Model file for the job. Use its own axes, mm. Face numbers are marked on the shaded views. A direction names the side the tool comes from. Round coordinates to 2 decimals unless told otherwise and drop trailing zeros. One line per item, written item: value.
from build123d import *

# Parameters (mm, degrees)
SKETCH1_R            = 4.1
BOSS_EXTRUDE1_DEPTH  = 6.35
SKETCH4_R            = 2
BOSS_EXTRUDE2_DEPTH  = 3
SKETCH6_R            = 1.999996081
BOSS_EXTRUDE4_DEPTH  = 3
SKETCH8_R            = 1.999996
BOSS_EXTRUDE5_DEPTH  = 3
SKETCH9_R            = 1.999996
BOSS_EXTRUDE6_DEPTH  = 3
SKETCH10_R           = 1.999996
BOSS_EXTRUDE7_DEPTH  = 3
SKETCH11_R           = 1.999996
BOSS_EXTRUDE8_DEPTH  = 3
SKETCH12_R           = 2.5
BOSS_EXTRUDE9_DEPTH  = 25.4
SKETCH15_R           = 5.5
SKETCH15_R_2         = 4
BOSS_EXTRUDE10_DEPTH = 2.54


with BuildPart() as part:
    # Sketch1 → Boss-Extrude1 (new body)
    with BuildSketch(Plane(origin=(0, 0, 0), x_dir=(1, 0, 0), z_dir=(0, 1, 0))):
        Polygon((1.878116929, -32.317100962), (-12.817952122, -29.725787478), (-10.907822168, -18.892902195), (3.788246884, -21.484215679), align=None)
        Polygon((-10.907822168, -18.892902195), (3.788246884, -21.484215679), (16.711753116, -14.022825876), (21.815644336, 0), (16.711753116, 14.022825876), (3.788246884, 21.484215679), (-10.907822168, 18.892902195), (-20.5, 7.461389802), (-20.5, -7.461389802), align=None)
        Circle(SKETCH1_R, mode=Mode.SUBTRACT)
        Polygon((27.048371945, 17.785047453), (32.152263164, 3.762221577), (21.815644336, 0), (16.711753116, 14.022825876), align=None)
        Polygon((-28.926488874, 14.532053509), (-19.334311042, 25.963565901), (-10.907822168, 18.892902195), (-20.5, 7.461389802), align=None)
    extrude(amount=BOSS_EXTRUDE1_DEPTH)

    # Sketch4 → Boss-Extrude2 (add)
    with BuildSketch(Plane(origin=(-5.469917597, 0, 31.02144422), x_dir=(-0.984807753, 0, -0.173648178), z_dir=(0.173648178, 0, -0.984807753))):
        with BuildLine():
            Line((-7.461389802, 6.35), (-7.461389802, 10.84999989))
            ThreePointArc((-7.461389802, 10.84999989), (0, 18.311389692), (7.461389802, 10.84999989))
            Line((7.461389802, 10.84999989), (7.461389802, 6.35))
            Line((7.461389802, 6.35), (-7.461389802, 6.35))
        make_face()
        with Locations((0, 10.84999989)):
            Circle(SKETCH4_R, mode=Mode.SUBTRACT)
    extrude(amount=BOSS_EXTRUDE2_DEPTH)

    # Sketch6 → Boss-Extrude4 (add)
    with BuildSketch(Plane(origin=(-3.559787642, 0, 20.188558937), x_dir=(-0.984807753, 0, -0.173648178), z_dir=(0.173648178, 0, -0.984807753))):
        with BuildLine():
            Line((-7.461389802, 6.35), (-7.461389802, 10.85))
            ThreePointArc((-7.461389802, 10.85), (0, 18.311389802), (7.461389802, 10.85))
            Line((7.461389802, 10.85), (7.461389802, 6.35))
            Line((7.461389802, 6.35), (-7.461389802, 6.35))
        make_face()
        with Locations((0, 10.85)):
            Circle(SKETCH6_R, mode=Mode.SUBTRACT)
    extrude(amount=-BOSS_EXTRUDE4_DEPTH)

    # Sketch8 → Boss-Extrude5 (add)
    with BuildSketch(Plane(origin=(29.600317555, 0, -10.773634515), x_dir=(0.342020143, 0, 0.939692621), z_dir=(-0.939692621, 0, 0.342020143))):
        with BuildLine():
            Line((-7.461389802, 10.85), (-7.461389802, 6.35))
            Line((-7.461389802, 6.35), (7.461389802, 6.35))
            Line((7.461389802, 6.35), (7.461389802, 10.85))
            ThreePointArc((7.461389802, 10.85), (0, 18.311389802), (-7.461389802, 10.85))
        make_face()
        with Locations((0, 10.85)):
            Circle(SKETCH8_R, mode=Mode.SUBTRACT)
    extrude(amount=BOSS_EXTRUDE5_DEPTH)

    # Sketch9 → Boss-Extrude6 (add)
    with BuildSketch(Plane(origin=(19.263698726, 0, -7.011412938), x_dir=(0.342020143, 0, 0.939692621), z_dir=(-0.939692621, 0, 0.342020143))):
        with BuildLine():
            Line((-7.461389802, 6.35), (-7.461389802, 10.85))
            ThreePointArc((-7.461389802, 10.85), (0, 18.311389802), (7.461389802, 10.85))
            Line((7.461389802, 10.85), (7.461389802, 6.35))
            Line((7.461389802, 6.35), (-7.461389802, 6.35))
        make_face()
        with Locations((0, 10.85)):
            Circle(SKETCH9_R, mode=Mode.SUBTRACT)
    extrude(amount=-BOSS_EXTRUDE6_DEPTH)

    # Sketch10 → Boss-Extrude7 (add)
    with BuildSketch(Plane(origin=(-24.130399958, 0, -20.247809705), x_dir=(0.64278761, 0, -0.766044443), z_dir=(0.766044443, 0, 0.64278761))):
        with BuildLine():
            Line((-7.461389802, 10.85), (-7.461389802, 6.35))
            Line((-7.461389802, 6.35), (7.461389802, 6.35))
            Line((7.461389802, 6.35), (7.461389802, 10.85))
            ThreePointArc((7.461389802, 10.85), (0, 18.311389802), (-7.461389802, 10.85))
        make_face()
        with Locations((0, 10.85)):
            Circle(SKETCH10_R, mode=Mode.SUBTRACT)
    extrude(amount=BOSS_EXTRUDE7_DEPTH)

    # Sketch11 → Boss-Extrude8 (add)
    with BuildSketch(Plane(origin=(-15.703911084, 0, -13.177145999), x_dir=(0.64278761, 0, -0.766044443), z_dir=(0.766044443, 0, 0.64278761))):
        with BuildLine():
            Line((-7.461389802, 10.85), (-7.461389802, 6.35))
            Line((-7.461389802, 6.35), (7.461389802, 6.35))
            Line((7.461389802, 6.35), (7.461389802, 10.85))
            ThreePointArc((7.461389802, 10.85), (0, 18.311389802), (-7.461389802, 10.85))
        make_face()
        with Locations((0, 10.85)):
            Circle(SKETCH11_R, mode=Mode.SUBTRACT)
    extrude(amount=-BOSS_EXTRUDE8_DEPTH)

    # Sketch12 → Boss-Extrude9 (add)
    with BuildSketch(Plane(origin=(0, 6.35, 0), x_dir=(1, 0, 0), z_dir=(0, 1, 0))):
        Polygon((16.711753116, -14.022825876), (17.976522258, -10.54790122), (16.711753116, -7.072976564), (13.50924523, -5.224007774), (9.867487631, -5.866147896), (7.490499173, -8.69893243), (7.490499173, -12.39687001), (9.867487631, -15.229654545), (13.50924523, -15.871794666), align=None)
        with Locations((12.570499173, -10.54790122)):
            Circle(SKETCH12_R, mode=Mode.SUBTRACT)
        Polygon((6.99075477, 12.685397576), (8.255523911, 16.160322233), (6.99075477, 19.635246889), (3.788246884, 21.484215679), (0.146489284, 20.842075557), (-2.230499173, 18.009291023), (-2.230499173, 14.311353442), (0.146489284, 11.478568908), (3.788246884, 10.836428786), align=None)
        with Locations((2.849500827, 16.160322233)):
            Circle(SKETCH12_R, mode=Mode.SUBTRACT)
        Polygon((-20.5, -7.461389802), (-18.123011542, -10.294174337), (-14.481253943, -10.936314459), (-11.278746057, -9.087345669), (-10.013976916, -5.612421012), (-11.278746057, -2.137496356), (-14.481253943, -0.288527566), (-18.123011542, -0.930667688), (-20.5, -3.763452222), align=None)
        with Locations((-15.42, -5.612421012)):
            Circle(SKETCH12_R, mode=Mode.SUBTRACT)
    extrude(amount=BOSS_EXTRUDE9_DEPTH)

    # Sketch15 → Boss-Extrude10 (add)
    with BuildSketch(Plane(origin=(0, 6.35, 0), x_dir=(1, 0, 0), z_dir=(0, 1, 0))):
        Circle(SKETCH15_R)
        Circle(SKETCH15_R_2, mode=Mode.SUBTRACT)
    extrude(amount=BOSS_EXTRUDE10_DEPTH)


solid = part.part
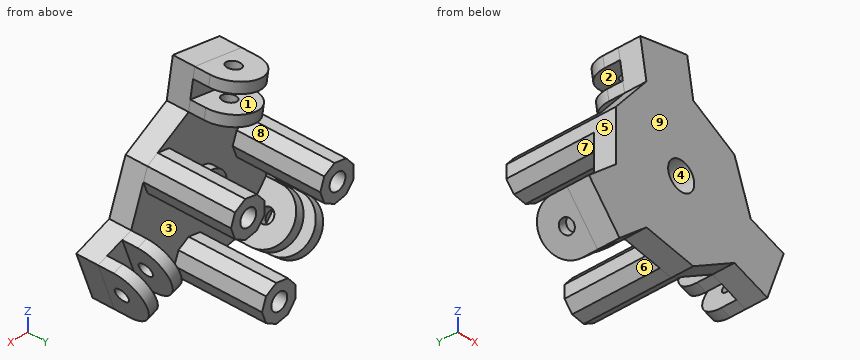
1. Mould opens along X. For the marked faces 1, 2, 3 and 4 say: released by +X, released by -X, zero draft, split by the parting line, or undercut.
Report:
face 1: released by -X
face 2: released by +X
face 3: undercut
face 4: undercut
2. Wall check: probe 1 along X at (y, z) = (16.5, -16.5); probe 2 along Z at (x, y) = (-14.5, 6.5); probe 3 along Y at (x, z) = (3.5, 7). Give the ranges that are in metal, low to high. Write a range as [from, to].
Report:
probe 1: [-27.25, -23.36], [-16.83, -12.92], [-2.23, 0.37], [5.33, 8.13]
probe 2: [-19.28, -14.61], [0.29, 3.29], [7.94, 10.93]
probe 3: [0, 6.35]
3. Drop flat-ended pins along their axis: pin 1 (4.5 mm diameter, centred on x = 2.85, z = -16.16, fed in from +Y); pin 2 (2 mm diameter, centred on y = 4.5, z = -6.5, fed in from -X); pin 3 (12 mm diameter, centred on x = -4.5, y = 4.5, fed in from +Z). Give the stop position or say it passes through.
Report:
pin 1: y = 6.35
pin 2: x = -20.55
pin 3: z = 32.25
4. Tool access for the marked faces 5, 6, 7, 8 and 9: list every direction of +Z, -Z, +X, -X, +Y, -Y with a clear straight run to the whole face (end or side of a thin tool).
Report:
face 5: +Z, -X, +Y, -Y
face 6: -Z, +Y
face 7: -X, +Y
face 8: +Y
face 9: +Z, -Z, +X, -X, -Y
5. Band-saw the part on A-A on y = 30. State how many separate pieces and enclosed holes the cut face has, plus the area to 3 significant figures.
Report:
separate pieces: 3
enclosed holes: 3
area: 195 mm²
